```python
from build123d import *

# Parameters (mm, degrees)
SKETCH1_W           = 8
SKETCH1_H           = 6
BOSS_EXTRUDE1_DEPTH = 4
SKETCH2_R           = 0.5
BOSS_EXTRUDE2_DEPTH = 6


with BuildPart() as part:
    # Sketch1 → Boss-Extrude1 (new body)
    with BuildSketch(Plane(origin=(0, 0, 0), x_dir=(1, 0, 0), z_dir=(0, 1, 0))):
        Rectangle(SKETCH1_W, SKETCH1_H)
    extrude(amount=BOSS_EXTRUDE1_DEPTH)

    # Sketch2 → Boss-Extrude2 (add, symmetric)
    with BuildSketch(Plane(origin=(0, 0, 0), x_dir=(0, 0, -1), z_dir=(1, 0, 0))):
        with Locations((-1, 2)):
            Circle(SKETCH2_R)
        with Locations((1, 2)):
            Circle(SKETCH2_R)
    extrude(amount=BOSS_EXTRUDE2_DEPTH, both=True)


solid = part.part
```
Check sheet for the modelled part. Datum: model origin and axes. Units: mm. A direction names the side the tool comes from. Round coordinates to 2 decimals unless told otherwise and drop trailing zeros. Order: outer loops, then holes, each group sorted by start corner. A loop starts at its lowest first (then second) coordinate and runs counter-clockwise, first axis right, second up. Notation, with made-up numbers: (72.25, -35) -> (122.25, -35) arc R19 cw to (122.25, -19) -> close; hole circle Ø11 at (55, 9.25). An arc over 180 degrees is marked (long way). One line per item, written item: value. Start each with the question number.
Q1. Set-up check for faces 4 (the face through (-4.986, 2.496, -0.935)), 5 (the face through (6, 2, 1)), 6 (the face through (4, 2, 0)): record each of +Z, -Z, +X, -X, +Y, -Y from which the full face is reachable in a straight line by a thin tool's end or side.
Q2. Cross-section at A-A (y = 2). Record the boundary of the cut face in (x, z).
Q3. Mould release check, pull along Z, two halves, no side actions. Record for faces 1 (the face through (0, 2, 3)), 2 (the face through (-6, 2, -1)), 3 (the face through (4.986, 2.496, 1.065)): pulls with the +Z half, pulls with the -Z half, needs draft (parallel to the pull), parting line crosses it, or undercut.
Q4. Cross-section at B-B (z = 1). Record the boundary of the cut face in (x, y).
Q5. Cross-section at C-C (x = 4.5). Record the boundary of the cut face in (y, z), and give its area (3 significant figures).
Q6. Thickness scan on line 1 (X direction, y = 0.8, z = 0.05); line 2 (Z direction, x = 4.5, y = 1.85); line 3 (Z direction, x = 4.5, y = 1.6). Record the ranges inside material, lowest first.
Completed:
1. face 4: -X
1. face 5: +Z, -Z, +X, +Y, -Y
1. face 6: +X
2. outline: (-6, -1.5) -> (-4, -1.5) -> (-4, -3) -> (4, -3) -> (4, -1.5) -> (6, -1.5) -> (6, -0.5) -> (4, -0.5) -> (4, 0.5) -> (6, 0.5) -> (6, 1.5) -> (4, 1.5) -> (4, 3) -> (-4, 3) -> (-4, 1.5) -> (-6, 1.5) -> (-6, 0.5) -> (-4, 0.5) -> (-4, -0.5) -> (-6, -0.5) -> close
3. face 1: pulls with the +Z half
3. face 2: needs draft
3. face 3: undercut
4. outline: (-6, 1.5) -> (-4, 1.5) -> (-4, 0) -> (4, 0) -> (4, 1.5) -> (6, 1.5) -> (6, 2.5) -> (4, 2.5) -> (4, 4) -> (-4, 4) -> (-4, 2.5) -> (-6, 2.5) -> close
5. outline: circle Ø1 at (2, -1); circle Ø1 at (2, 1)
5. area: 1.57 mm²
6. line 1: x = -4 to 4
6. line 2: z = -1.48 to -0.52, 0.52 to 1.48
6. line 3: z = -1.3 to -0.7, 0.7 to 1.3
